Work out the finished part from the listing and answer in its coordinate system (mm). A direction names the side the tool comes from. Coordinates: 2 decimals unless noted, no trailing zeros. Loops run counter-clockwise (first coordinate to the right, second up) from the corner with the lowest first, then second, coordinate; pieces in that order, holes last. Notation, with made-up numbers: (71.5, 69) - (128.5, 69) arc R12 ccw to (128.5, 77) - close; hole circle Ø9 at (20, 77.5). An arc over 180 degrees is marked (long way). Write each question's results on one line, items separated by ' | '. Start each with the question number.
Item 1: Each of these flat-tipped pins is pushed along its axis until it touches: pin 1 Ø2 at (x, y) = (-29, 1.5) entering from -Z; pin 2 Ø2 at (y, z) = (3.5, -26.5) entering from +X; pin 3 Ø9.5 at (x, z) = (-43, 0) entering from -Y; pin 4 Ø5 at (x, z) = (-30, -1) entering from +Y. Where does it stop, or does it pass through?
Item 2: Section C-C, the plane z = -43 is taken. Write down the section's boundary in (x, y), plus the area to 3 significant figures.
Item 3: Consider probe 1 along X at (y, z) = (7.4, 0); probe 2 along X at (y, z) = (4, 0); probe 3 along X at (y, z) = (4.85, 0). Determine where each line is inside the solid, lowest interval first. Write a range as [from, to].
Item 4: Section D-D, the plane x = -43 is taken. Write down the section's boundary in (y, z).
Item 5: Section A-A, the plane y = 1.75 is taken. Write down the section's boundary in (x, z).
Item 6: Section B-B, the plane x = 0 is taken. Write down the section's boundary in (y, z).
Item 7: A tool of negligible diameter and unlimited length cuts with its end or side. For faces 5 (the face through (38.904, 4.056, -0.18)), 6 (the face through (-27, 2, -5.05)), 7 (the face through (15, 6, 15)), from which of +Z, -Z, +X, -X, +Y, -Y can it reach the whole face along a straight path? Write none if from no direction.
Item 8: For a pull along X with two mould halves and no side action, classify faces 1 (the face through (-15, 8, 33)), 2 (the face through (-31.296, 5.162, 0.167)), 3 (the face through (47.69, 3.94, -15.02)), 4 (the face through (-31.853, 2.12, -2.56)) as +X half, -X half, draft (parallel to the pull), parting line (faces both ways), or undercut.
from build123d import *

# Parameters (mm, degrees)
SKETCH1_R               = 50
SKETCH1_R_2             = 35.5
BOSS_EXTRUDE1_DEPTH     = 8
SKETCH2_R               = 4.1
CUT_EXTRUDE1_DEPTH      = 1
CUT_EXTRUDE1_DEPTH_BACK = 9
SKETCH3_R               = 35.5
SKETCH3_R_2             = 20
BOSS_EXTRUDE2_DEPTH     = 6
CUT_EXTRUDE2_START      = -6
CUT_EXTRUDE2_DEPTH      = 4.3
SKETCH5_R               = 3.8
CUT_EXTRUDE3_DEPTH      = 7
CUT_EXTRUDE3_DEPTH_BACK = 3


with BuildPart() as part:
    # Sketch1 → Boss-Extrude1 (new body)
    with BuildSketch(Plane(origin=(0, 0, 0), x_dir=(1, 0, 0), z_dir=(0, 1, 0))):
        Circle(SKETCH1_R)
        Circle(SKETCH1_R_2, mode=Mode.SUBTRACT)
    extrude(amount=BOSS_EXTRUDE1_DEPTH)

    # Sketch2 → Cut-Extrude1 (cut, two sides)
    with BuildSketch(Plane(origin=(0, 8, 0), x_dir=(1, 0, 0), z_dir=(0, 1, 0))) as cut_extrude1_sk:
        with Locations((0, -43)):
            Circle(SKETCH2_R)
        with Locations((-43, 0)):
            Circle(SKETCH2_R)
        with Locations((0, 43)):
            Circle(SKETCH2_R)
        with Locations((43, 0)):
            Circle(SKETCH2_R)
    extrude(amount=CUT_EXTRUDE1_DEPTH, mode=Mode.SUBTRACT)
    extrude(cut_extrude1_sk.sketch, amount=-CUT_EXTRUDE1_DEPTH_BACK, mode=Mode.SUBTRACT)

    # Sketch3 → Boss-Extrude2 (add)
    with BuildSketch(Plane(origin=(0, 0, 0), x_dir=(1, 0, 0), z_dir=(0, 1, 0))):
        Circle(SKETCH3_R)
        Circle(SKETCH3_R_2, mode=Mode.SUBTRACT)
    extrude(amount=BOSS_EXTRUDE2_DEPTH)

    # Sketch4 → Cut-Extrude2 (cut)
    with BuildSketch(Plane(origin=(0, 6, 0), x_dir=(1, 0, 0), z_dir=(0, 1, 0)).offset(CUT_EXTRUDE2_START)):
        Polygon((-21.668762281, 0), (-24.584381141, 5.05), (-30.415618859, 5.05), (-33.331237719, 0), (-30.415618859, -5.05), (-24.584381141, -5.05), align=None)
        Polygon((33.331237719, 0), (30.415618859, 5.05), (24.584381141, 5.05), (21.668762281, 0), (24.584381141, -5.05), (30.415618859, -5.05), align=None)
    extrude(amount=CUT_EXTRUDE2_DEPTH, mode=Mode.SUBTRACT)

    # Sketch5 → Cut-Extrude3 (cut, two sides)
    with BuildSketch(Plane(origin=(0, 6, -6), x_dir=(1, 0, 0), z_dir=(0, -1, 0))) as cut_extrude3_sk:
        with Locations((-27.5, 6)):
            Circle(SKETCH5_R)
        with Locations((27.5, 6)):
            Circle(SKETCH5_R)
    extrude(amount=CUT_EXTRUDE3_DEPTH, mode=Mode.SUBTRACT)
    extrude(cut_extrude3_sk.sketch, amount=-CUT_EXTRUDE3_DEPTH_BACK, mode=Mode.SUBTRACT)


solid = part.part
Answer key:
1) pin 1: stops at z = -41.42 | pin 2: stops at x = 43.01 | pin 3: stops at y = 0 | pin 4: stops at y = 6
2) outline: (-25.51, 0) - (-4.1, 0) - (-4.1, 8) - (-25.51, 8) - close; (4.1, 0) - (25.51, 0) - (25.51, 8) - (4.1, 8) - close | area: 343 mm^2
3) probe 1: x = [-50, -47.1], [-38.9, -35.5], [35.5, 38.9], [47.1, 50] | probe 2: x = [-50, -47.1], [-38.9, -33.33], [-21.67, -20], [20, 21.67], [33.33, 38.9], [47.1, 50] | probe 3: x = [-50, -47.1], [-38.9, -31.3], [-23.7, -20], [20, 23.7], [31.3, 38.9], [47.1, 50]
4) outline: (0, -25.51) - (8, -25.51) - (8, -4.1) - (0, -4.1) - close; (0, 4.1) - (8, 4.1) - (8, 25.51) - (0, 25.51) - close
5) outline: circle Ø100 at (0, 0); hole circle Ø8.2 at (-43, 0); hole (-33.33, 0) - (-30.42, -5.05) - (-24.58, -5.05) - (-21.67, 0) - (-24.58, 5.05) - (-30.42, 5.05) - close; hole circle Ø40 at (0, 0); hole circle Ø8.2 at (0, -43); hole circle Ø8.2 at (0, 43); hole (21.67, 0) - (24.58, -5.05) - (30.42, -5.05) - (33.33, 0) - (30.42, 5.05) - (24.58, 5.05) - close; hole circle Ø8.2 at (43, 0)
6) outline: (0, -50) - (8, -50) - (8, -47.1) - (0, -47.1) - close; (0, -38.9) - (8, -38.9) - (8, -35.5) - (6, -35.5) - (6, -20) - (0, -20) - close; (0, 20) - (6, 20) - (6, 35.5) - (8, 35.5) - (8, 38.9) - (0, 38.9) - close; (0, 47.1) - (8, 47.1) - (8, 50) - (0, 50) - close
7) face 5: +Y, -Y | face 6: -Y | face 7: +Y
8) face 1: draft | face 2: undercut | face 3: parting line | face 4: undercut
